Work out the finished part from the listing and answer in its coordinate system (mm). A direction names the side the tool comes from. Coordinates: 2 decimals unless noted, no trailing zeros. Loops run counter-clockwise (first coordinate to the right, second up) from the corner with the lowest first, then second, coordinate; pieces in that order, holes last. Notation, with made-up numbers: (-39, 78) -> (-11, 78) arc R18 ccw to (-11, 103) -> close; hole circle Ø4 at (48, 13.5). An arc over 180 degrees is marked (long way). Answer as CSV lines item,"result".
```python
from build123d import *

# Parameters (mm, degrees)
SKETCH_1_R          = 1.25
EXTRUDE_1_DEPTH     = 5
SKETCH_2_W          = 5
SKETCH_2_H          = 25
EXTRUDE_2_DEPTH     = 4
SKETCH_3_W          = 4
SKETCH_3_H          = 25
EXTRUDE_3_DEPTH     = 20
SKETCH_4_R          = 1.5
CUT_EXTRUDE_1_DEPTH = 20
EXTRUDE_START       = -5
SKETCH_7_R          = 1.25
EXTRUDE_4_DEPTH     = 5
SKETCH_8_R          = 1.5
SKETCH_8_R_2        = 4
EXTRUDE_5_DEPTH     = 5
EXTRUDE_START_2     = 4
SKETCH_14_W         = 25
SKETCH_14_H         = 25
SKETCH_14_R         = 1.5
EXTRUDE_9_DEPTH     = 4
SKETCH_15_W         = 4
SKETCH_15_H         = 25
CUT_EXTRUDE_2_DEPTH = 100
SKETCH_19_W         = 1.750049733
SKETCH_19_H         = 25
EXTRUDE_10_DEPTH    = 20
SKETCH_20_R         = 1.5
CUT_EXTRUDE_3_DEPTH = 20
SKETCH_21_W         = 25
SKETCH_21_H         = 25
CUT_EXTRUDE_4_DEPTH = 4
SKETCH_22_W         = 1.750049733
SKETCH_22_H         = 25
EXTRUDE_11_DEPTH    = 5


with BuildPart() as part:
    # 草图1 → 凸台-拉伸1 (new body)
    with BuildSketch(Plane.XY):
        Polygon((-3.581151343, -8.027992706), (-3.581151343, -12.611885422), (2.918848657, -12.611885422), (2.918848657, -6.641886627), (2.918848657, 12.388114578), (-3.581151343, 12.388114578), align=None)
        with Locations((-0.081151343, 8.237522913)):
            Circle(SKETCH_1_R, mode=Mode.SUBTRACT)
        with Locations((-0.081151343, 2.787522913)):
            Circle(SKETCH_1_R, mode=Mode.SUBTRACT)
        with Locations((-0.081151343, -2.662477087)):
            Circle(SKETCH_1_R, mode=Mode.SUBTRACT)
        with Locations((-0.000846901, -8.111885422)):
            Circle(SKETCH_1_R, mode=Mode.SUBTRACT)
    extrude(amount=EXTRUDE_1_DEPTH)

    # 草图2 → 凸台-拉伸2 (add)
    with BuildSketch(Plane.ZY.offset(3.581151343)):
        with Locations((2.5, -0.111885422)):
            Rectangle(SKETCH_2_W, SKETCH_2_H)
    extrude(amount=EXTRUDE_2_DEPTH)

    # 草图3 → 凸台-拉伸3 (add)
    with BuildSketch(Plane(origin=(0, 0, 0), x_dir=(-1, 0, 0), z_dir=(0, 0, -1))):
        with Locations((5.581151343, -0.111885422)):
            Rectangle(SKETCH_3_W, SKETCH_3_H)
    extrude(amount=EXTRUDE_3_DEPTH)

    # 草图4 → 切除-拉伸1 (cut)
    with BuildSketch(Plane(origin=(-3.581151343, 0, 0), x_dir=(0, 0, -1), z_dir=(1, 0, 0))):
        with Locations(Location((6, 3.388114578, 0), (0, 0, 90))):
            Circle(SKETCH_4_R)
        with Locations(Location((14, 3.388114578, 0), (0, 0, 180))):
            Circle(SKETCH_4_R)
        with Locations(Location((14, -4.611885422, 0), (0, 0, 90))):
            Circle(SKETCH_4_R)
        with Locations(Location((6, -4.611885422, 0), (0, 0, 180))):
            Circle(SKETCH_4_R)
    extrude(amount=-CUT_EXTRUDE_1_DEPTH, mode=Mode.SUBTRACT)

    # 草图7 → 凸台-拉伸4 (add)
    with BuildSketch(Plane.XY.offset(5).offset(EXTRUDE_START)):
        with Locations((-0.081151343, 8.237522913)):
            Circle(SKETCH_7_R)
        with Locations((-0.081151343, 2.787522913)):
            Circle(SKETCH_7_R)
        with Locations((-0.081151343, -2.662477087)):
            Circle(SKETCH_7_R)
        with Locations((-0.000846901, -8.111885422)):
            Circle(SKETCH_7_R)
    extrude(amount=EXTRUDE_4_DEPTH)

    # 草图8 → 凸台-拉伸5 (add)
    with BuildSketch(Plane.XY.offset(5)):
        with BuildLine():
            ThreePointArc((9.045368421, 28.911309576), (-0.331303735, 42.388418969), (-9.707833242, 28.911210329))
            Line((-9.707833242, 28.911210329), (-3.581151343, 12.388114578))
            Line((-3.581151343, 12.388114578), (2.918848657, 12.388114578))
            Line((2.918848657, 12.388114578), (9.045368421, 28.911309576))
        make_face()
        with Locations((-0.33125081, 25.388000558)):
            Circle(SKETCH_8_R, mode=Mode.SUBTRACT)
        with Locations((-7.33125081, 32.388000558)):
            Circle(SKETCH_8_R, mode=Mode.SUBTRACT)
        with Locations((-0.33125081, 32.388000558)):
            Circle(SKETCH_8_R_2, mode=Mode.SUBTRACT)
        with Locations((-0.33125081, 39.388000558)):
            Circle(SKETCH_8_R, mode=Mode.SUBTRACT)
        with Locations((6.668848657, 32.388114578)):
            Circle(SKETCH_8_R, mode=Mode.SUBTRACT)
    extrude(amount=-EXTRUDE_5_DEPTH)

    # 草图14 → 凸台-拉伸9 (add)
    with BuildSketch(Plane(origin=(2.918848657, 0, 0), x_dir=(0, 0, -1), z_dir=(1, 0, 0)).offset(EXTRUDE_START_2)):
        with Locations((7.5, -0.111885422)):
            Rectangle(SKETCH_14_W, SKETCH_14_H)
        with Locations(Location((6, 3.388114578, 0), (0, 0, 90))):
            Circle(SKETCH_14_R, mode=Mode.SUBTRACT)
        with Locations(Location((14, 3.388114578, 0), (0, 0, 180))):
            Circle(SKETCH_14_R, mode=Mode.SUBTRACT)
        with Locations(Location((14, -4.611885422, 0), (0, 0, 90))):
            Circle(SKETCH_14_R, mode=Mode.SUBTRACT)
        with Locations(Location((6, -4.611885422, 0), (0, 0, 180))):
            Circle(SKETCH_14_R, mode=Mode.SUBTRACT)
    extrude(amount=-EXTRUDE_9_DEPTH)

    # 草图15 → 切除-拉伸2 (cut)
    with BuildSketch(Plane(origin=(0, 0, -20), x_dir=(-1, 0, 0), z_dir=(0, 0, -1))):
        with Locations((5.581151343, -0.111885422)):
            Rectangle(SKETCH_15_W, SKETCH_15_H)
    extrude(amount=-CUT_EXTRUDE_2_DEPTH, mode=Mode.SUBTRACT)

    # 草图19 → 凸台-拉伸10 (add)
    with BuildSketch(Plane(origin=(0, 0, 0), x_dir=(-1, 0, 0), z_dir=(0, 0, -1))):
        with Locations((4.45617621, -0.111885422)):
            Rectangle(SKETCH_19_W, SKETCH_19_H)
        Polygon((1.331201076, 12.388114578), (1.331201076, 9.888057568), (1.331201076, -12.611885422), (3.581151343, -12.611885422), (3.581151343, 12.388114578), align=None)
    extrude(amount=EXTRUDE_10_DEPTH)

    # 草图20 → 切除-拉伸3 (cut)
    with BuildSketch(Plane(origin=(6.918848657, 0, 0), x_dir=(0, 0, -1), z_dir=(1, 0, 0))):
        with Locations(Location((6, 3.388114578, 0), (0, 0, 90))):
            Circle(SKETCH_20_R)
        with Locations(Location((14, 3.388114578, 0), (0, 0, 90))):
            Circle(SKETCH_20_R)
        with Locations(Location((6, -4.611885422, 0), (0, 0, 90))):
            Circle(SKETCH_20_R)
        with Locations(Location((14, -4.611885422, 0), (0, 0, 90))):
            Circle(SKETCH_20_R)
    extrude(amount=-CUT_EXTRUDE_3_DEPTH, mode=Mode.SUBTRACT)

    # 草图21 → 切除-拉伸4 (cut)
    with BuildSketch(Plane(origin=(6.918848657, 0, 0), x_dir=(0, 0, -1), z_dir=(1, 0, 0))):
        with Locations((7.5, -0.111885422)):
            Rectangle(SKETCH_21_W, SKETCH_21_H)
    extrude(amount=-CUT_EXTRUDE_4_DEPTH, mode=Mode.SUBTRACT)

    # 草图22 → 凸台-拉伸11 (add)
    with BuildSketch(Plane.XY):
        with Locations((-4.45617621, -0.111885422)):
            Rectangle(SKETCH_22_W, SKETCH_22_H)
    extrude(amount=EXTRUDE_11_DEPTH)


solid = part.part
```
(1) A cutting plane is placed at A-A, the plane x = -2.5. Write down the section's boundary in (y, z), and give its area (3 significant figures).
Computed values:
outline,"(-12.61, -20) -> (12.39, -20) -> (12.39, 0) -> (29.03, 0) -> (29.03, 5) -> (-12.61, 5) -> close; (35.75, 0) -> (42.15, 0) -> (42.15, 5) -> (35.75, 5) -> close; hole circle Ø3 at (-4.61, -14); hole circle Ø3 at (-4.61, -6); hole circle Ø3 at (3.39, -14); hole circle Ø3 at (3.39, -6)"
area,"712 mm2"
(2) For a pull along Z with two mould halves and no side action, classify faces 1 (the face through (0, 21, 0)), 2 (the face through (-3.303, 4.774, -6.575)), 3 (the face through (-3, -12.612, -5)) as pulls with the +Z half, pulls with the -Z half, needs draft (parallel to the pull), parting line crosses it, or undercut.
Computed values:
face 1,"pulls with the -Z half"
face 2,"undercut"
face 3,"needs draft"
(3) A cutting plane is placed at D-D, the plane y = 10.5. Write down the section's boundary in (x, z), and give its area (3 significant figures).
Computed values:
outline,"(-5.33, -20) -> (-1.33, -20) -> (-1.33, 0) -> (2.92, 0) -> (2.92, 5) -> (-5.33, 5) -> close"
area,"121 mm2"
(4) A cutting plane is placed at C-C, the plane y = 3. Write down the section's boundary in (x, z).
Computed values:
outline,"(-5.33, -20) -> (-1.33, -20) -> (-1.33, -15.45) -> (-5.33, -15.45) -> close; (-5.33, -12.55) -> (-1.33, -12.55) -> (-1.33, -7.45) -> (-5.33, -7.45) -> close; (-5.33, -4.55) -> (-1.33, -4.55) -> (-1.33, 0) -> (2.92, 0) -> (2.92, 5) -> (-5.33, 5) -> close"
(5) A cutting plane is placed at B-B, the plane z = -6. Write down the section's boundary in (x, y), and give its area (3 significant figures).
Computed values:
outline,"(-5.33, -12.61) -> (-1.33, -12.61) -> (-1.33, -6.11) -> (-5.33, -6.11) -> close; (-5.33, -3.11) -> (-1.33, -3.11) -> (-1.33, 1.89) -> (-5.33, 1.89) -> close; (-5.33, 4.89) -> (-1.33, 4.89) -> (-1.33, 12.39) -> (-5.33, 12.39) -> close"
area,"76.0 mm2"
(6) Flat-ended cylindrical pins translate along their axes: pin 1 Ø2.5 at (x, y) = (-7.33, 32.39) entering from -Z; pin 2 Ø3 at (y, z) = (-4.5, -17) entering from +X; pin 3 Ø4 at (y, z) = (6.5, -16.5) entering from -X; pin 4 Ø10 at (x, y) = (-1, 12.5) entering from -Z. Find the tip coordinate at first contact, or state that the pin passes through.
Computed values:
pin 1,"through"
pin 2,"x = -1.33"
pin 3,"x = -5.33"
pin 4,"z = -20"
(7) Consider line 1 along Z through (x, y) = (-4, 16.5); line 2 along Y through (x, z) = (-1.5, 4); line 3 along X through (y, z) = (7, -13.75). Determine where each line is inside the solid, lowest interval first.
Computed values:
line 1,"0 to 5"
line 2,"-12.61 to 24.45, 26.33 to 28.56, 36.21 to 38.45, 40.33 to 42.32"
line 3,"-5.33 to -1.33"
(8) Which of the six approach directions +Z, -Z, +X, -X, +Y, -Y give full straight-line access (tool end or side, diameter ignored) to faces 4 (the face through (-6.7, 20.8, 2.5)), 5 (the face through (0, 15, 5)), 6 (the face through (-5.331, 0, -8)), 7 (the face through (-1.331, 0, -10)), 8 (the face through (2.919, 0, 3))?
Computed values:
face 4,"+Z, -Z, -X"
face 5,"+Z, +X, -X, +Y, -Y"
face 6,"+Z, -Z, -X, -Y"
face 7,"-Z, +X, +Y, -Y"
face 8,"+Z, -Z, +X, -Y"
